from build123d import *

# Parameters (mm, degrees)
EXTRUDE_1_DEPTH     = 3
SKETCH_2_R          = 1.3
CUT_EXTRUDE_1_DEPTH = 4


with BuildPart() as part:
    # 스케치1 → 보스-돌출1 (new body)
    with BuildSketch(Plane.XY):
        with BuildLine():
            ThreePointArc((5.908095924, 12.125440592), (-2.734946833, 7.908149395), (-6.618010934, -0.890120111))
            ThreePointArc((-6.618010934, -0.890120111), (-3.819295692, -4.078723723), (-0.63069208, -1.280008481))
            ThreePointArc((-0.63069208, -1.280008481), (1.675267899, 3.836644085), (6.775226967, 6.179292672))
            ThreePointArc((6.775226967, 6.179292672), (26.056169451, 4.379851204), (43.709409242, -3.57978808))
            ThreePointArc((43.709409242, -3.57978808), (47.849012899, -2.782847709), (47.104702299, 1.366541899))
            ThreePointArc((47.104702299, 1.366541899), (27.481967947, 10.481515342), (5.908095924, 12.125440592))
        make_face()
    extrude(amount=EXTRUDE_1_DEPTH)

    # 스케치2 → 컷-돌출1 (cut, through all)
    with BuildSketch(Plane.XY.offset(3)):
        with Locations((-3.624351507, -1.085064296)):
            Circle(SKETCH_2_R)
        with Locations((45.375648493, -1.085064296)):
            Circle(SKETCH_2_R)
    extrude(amount=-CUT_EXTRUDE_1_DEPTH, mode=Mode.SUBTRACT)


solid = part.part
Input: part model. Units: mm. Frame: model coordinates. A direction names the side the tool comes from. Round coordinates to 2 decimals unless told otherwise and drop trailing zeros. Order: outer loops, then holes, each group sorted by start corner. A loop starts at its lowest first (then second) coordinate and runs counter-clockwise, first axis right, second up. Notation, with made-up numbers: (28.25, 65.25) - (34.25, 65.25) arc R17 ccw to (34.25, 85.25) - close; hole circle Ø1 at (14, 63). An arc over 180 degrees is marked (long way). Use a Markdown table: item, result.
1. Section B-B on z = 1.1. Return the cut outline in (x, y), then the cut area to 3 significant figures.
Evaluation:
| item | result |
|---|---|
| outline | (-6.62, -0.89) arc R3 ccw to (-0.63, -1.28) arc R8 cw to (6.78, 6.18) arc R58.85 cw to (43.71, -3.58) arc R3 ccw to (47.1, 1.37) arc R60.63 ccw to (5.91, 12.13) arc R14 ccw to start; hole circle Ø2.6 at (-3.62, -1.09); hole circle Ø2.6 at (45.38, -1.09) |
| area | 365 mm^2 |
2. Section C-C on x = 33. Return the cut outline in (y, z), then the cut area to 3 significant figures.
Evaluation:
| item | result |
|---|---|
| outline | (2.07, 0) - (8.76, 0) - (8.76, 3) - (2.07, 3) - close |
| area | 20.0 mm^2 |
3. Section D-D on y = 9.5. Return the cut outline in (x, z).
Evaluation:
| item | result |
|---|---|
| outline | (-0.91, 0) - (30.84, 0) - (30.84, 3) - (-0.91, 3) - close |
4. Mould query, pull axis X, two halves, no side actions, for faces 3 (the face through (-2.639, 8.007, 1.479)), 4 (the face through (-3.906, -2.354, 1.521)), 5 (the face through (20, 6, 3)). Classes: +X half, -X half, draft (parallel to the pull), parting line (faces both ways), or undercut.
Evaluation:
| item | result |
|---|---|
| face 3 | -X half |
| face 4 | undercut |
| face 5 | draft |
5. First-contact query: pin 1 (1.6 mm diameter, centred on x = 45.38, y = -1.09, fed in from +Z). Flat tip, straight axial feed; report the tip coordinate or a pass-through.
Evaluation:
| item | result |
|---|---|
| pin 1 | through |
6. Material intervals for probe 1 along X at (y, z) = (-1.5, 2.6); probe 2 along X at (y, z) = (-0.25, 1.4); probe 3 along Y at (x, z) = (45, 1.55), sorted ascending.
Evaluation:
| item | result |
|---|---|
| probe 1 | -6.6 to -4.86, -2.39 to -0.65, 40.36 to 44.14, 46.61 to 48.35 |
| probe 2 | -6.56 to -4.62, -2.63 to -0.5, 38.07 to 44.38, 46.37 to 48.26 |
| probe 3 | -4.06 to -2.33, 0.16 to 2.79 |
7. Section A-A on y = 2.5. Return the cut outline in (x, z).
Evaluation:
| item | result |
|---|---|
| outline | (-5.97, 0) - (0.61, 0) - (0.61, 3) - (-5.97, 3) - close; (31.91, 0) - (45.44, 0) - (45.44, 3) - (31.91, 3) - close |
8. Access query for faces 1 (the face through (20, 6, 0)), 2 (the face through (1.62, 3.78, 1.48)). Directions: +Z, -Z, +X, -X, +Y, -Y. A direction counts if a zero-diameter tool reaches every point of the face in a straight line with its end or side. Return the directions, or none.
Evaluation:
| item | result |
|---|---|
| face 1 | -Z, +X, -X, +Y, -Y |
| face 2 | +Z, -Z, -Y |
